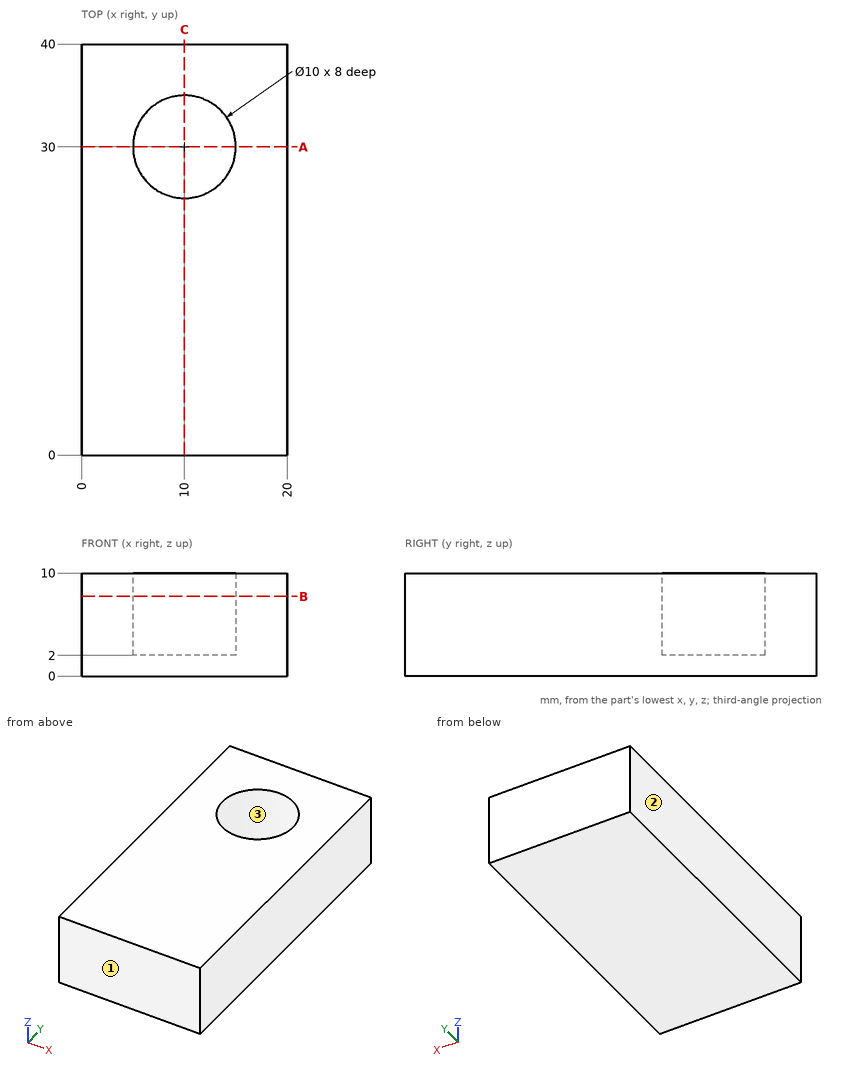
Geometry check sheet. Reference: drawing and pictorial views, mm from the part's lowest x, y, z. Round coordinates to 2 decimals unless told otherwise and drop trailing zeros. Loops run counter-clockwise (first coordinate to the right, second up) from the corner with the lowest first, then second, coordinate; pieces in that order, holes last.
1. Sectioned sample at B-B on z = 7.75. Record the boundary of the cut face in (x, y), and give its area (3 significant figures).
2. Sectioned sample at C-C on x = 10. Record the boundary of the cut face in (y, z), and give its area (3 significant figures).
3. Gauge pin test, flat ends, axial feed: pin 1 Ø3 at (x, y) = (11, 32.5) entering from +Z; pin 2 Ø6 at (x, y) = (10, 35) entering from -Z. Record the tip position at first contact, or that the pin passes through.
4. Mould release check, pull along Y, two halves, no side actions. Record for the marked faces 1, 2 and 3: released by +Y, released by -Y, zero draft, split by the parting line, or undercut.
5. Sectioned sample at A-A on y = 30. Record the boundary of the cut face in (x, z), and give its area (3 significant figures).
6. Scan lines: probe 1 along Y at (x, z) = (10, 5.5); probe 2 along X at (y, z) = (30.5, 7); probe 3 along Z at (x, y) = (12, 29). Record each from-to range of solid material in increasing order.
Recorded:
1. outline: (0, 0) - (20, 0) - (20, 40) - (0, 40) - close; hole circle Ø10 at (10, 30)
1. area: 721 mm2
2. outline: (0, 0) - (40, 0) - (40, 10) - (35, 10) - (35, 2) - (25, 2) - (25, 10) - (0, 10) - close
2. area: 320 mm2
3. pin 1: stops at z = 2
3. pin 2: stops at z = 0
4. face 1: released by -Y
4. face 2: zero draft
4. face 3: undercut
5. outline: (0, 0) - (20, 0) - (20, 10) - (15, 10) - (15, 2) - (5, 2) - (5, 10) - (0, 10) - close
5. area: 120 mm2
6. probe 1: y = 0 to 25, 35 to 40
6. probe 2: x = 0 to 5.03, 14.97 to 20
6. probe 3: z = 0 to 2
